```python
from build123d import *

# Parameters (mm, degrees)
F0_W     = 25
F0_H     = 50
F1_DEPTH = 75
F2_DEPTH = 50
F3_DEPTH = 75


with BuildPart() as f1:
    # F0 (on Top) → F1 (new body)
    with BuildSketch(Plane.XY):
        with Locations((12.5, 25)):
            Rectangle(F0_W, F0_H)
    extrude(amount=F1_DEPTH)

    # F0 (on Top) → F2 (join)
    with BuildSketch(Plane.XY):
        Polygon((25, 50), (25, 0), (42.5, 0), (42.5, 10), (70, 10), (70, 5), (95, 5), (95, 50), (70, 50), (42.5, 50), align=None)
    extrude(amount=F2_DEPTH)

    # F0 (on Top) → F3 (join)
    with BuildSketch(Plane.XY):
        Polygon((125, 50), (95, 50), (95, 5), (105, 5), (105, -20), (125, -20), (125, 5), align=None)
    extrude(amount=F3_DEPTH)


solid = f1.part
```
Geometry: final body of the model. Coordinates: model frame, mm. A direction names the side the tool comes from. Give positions to 0.01 mm unless a question says otherwise; leave off trailing zeros. Write each loop counter-clockwise with the first axis right and the second up, starting at its lowest first coordinate (ties: lowest second). Pieces come first, ordered by that corner, then holes.
1. Section query A-A, the plane y = 1.5. Return loops of the section in (x, z), then the cut area to 3 significant figures.
2. Section query C-C, the plane z = 30.5. Return loops of the section in (x, y), then the cut area to 3 significant figures.
3. Reachability of faces 1 (the flat face through (0, 25, 37)), 2 (the flat face through (105, -7, 37)), 3 (the flat face through (60, 31, 50)) from +Z, -Z, +X, -X, +Y, -Y: full face, straight path, thin tool, end or side. Return the list, or none.
4. Line query: probe 1 along X at (y, z) = (10.5, 63); probe 2 along Y at (x, z) = (77, 18); probe 3 along X at (y, z) = (-8, 60.5). Output: solid intervals per line, ascending.
5. Section query D-D, the plane y = 21.5. Return loops of the section in (x, z).
6. Draft query along X for faces 4 (the flat face through (70, 8, 25)), 5 (the flat face through (21, 0, 29)), 6 (the flat face through (125, 15, 37)), 7 (the flat face through (87, 5, 29)). Return one class per face: released by +X, released by -X, zero draft, split by the parting line, or undercut.
7. Pin query (flat end, axial travel): P1, Ø5, axis at x = 100.5, z = 49.5, coming from the -Y side; P2, Ø8, axis at x = 54, z = 34, coming from the -Y side; P3, Ø21, axis at x = 28.5, z = 54, coming from the -Y side. Return the tip coordinate at first contact, or that it passes through.
8. Section query B-B, the plane z = 56. Return loops of the section in (x, y).
Computed:
1. outline: (0, 0) - (42.5, 0) - (42.5, 50) - (25, 50) - (25, 75) - (0, 75) - close; (105, 0) - (125, 0) - (125, 75) - (105, 75) - close
1. area: 4,250 mm2
2. outline: (0, 0) - (42.5, 0) - (42.5, 10) - (70, 10) - (70, 5) - (105, 5) - (105, -20) - (125, -20) - (125, 50) - (0, 50) - close
2. area: 6,200 mm2
3. face 1: +Z, -Z, -X, +Y, -Y
3. face 2: +Z, -Z, -Y
3. face 3: +Z, +Y, -Y
4. probe 1: x = 0 to 25, 95 to 125
4. probe 2: y = 5 to 50
4. probe 3: x = 105 to 125
5. outline: (0, 0) - (125, 0) - (125, 75) - (95, 75) - (95, 50) - (25, 50) - (25, 75) - (0, 75) - close
6. face 4: undercut
6. face 5: zero draft
6. face 6: released by +X
6. face 7: undercut
7. P1: stops at y = 5
7. P2: stops at y = 10
7. P3: stops at y = 0
8. outline: (0, 0) - (25, 0) - (25, 50) - (0, 50) - close; (95, 5) - (105, 5) - (105, -20) - (125, -20) - (125, 50) - (95, 50) - close
